Input: part model. Units: mm. Frame: model coordinates. Round coordinates to 2 decimals unless told otherwise and drop trailing zeros. Order: outer loops, then holes, each group sorted by start corner. A loop starts at its lowest first (then second) coordinate and runs counter-clockwise, first axis right, second up. Notation, with made-up numbers: M 27,84 L 58,84 A31 cw 58,118 Z; hole C -25.75,-29.75 d8. An arc over 180 degrees is marked long. One line per question, with ' | ' between items.
Autodesk Inventor part; units mm, degrees
ref_plane "YZ Plane" through (0, 0, 0) normal (1, 0, 0) x (0, 1, 0)
ref_plane "XZ Plane" through (0, 0, 0) normal (0, 1, 0) x (-1, 0, 0)
ref_plane "XY Plane" through (0, 0, 0) normal (0, 0, 1) x (1, 0, 0)
sketch "Esquisse1" plane through (0, 0, 0) normal (0, 0, 1) x (1, 0, 0)
  line L0 (22.3904, 80.6375) -> (22.3904, -39.3625)
  line L1 (-37.6096, 80.6375) -> (-37.6096, -39.3625)
  line L2 (-37.6096, -39.3625) -> (22.3904, -39.3625)
  line L3 (-37.6096, 80.6375) -> (22.3904, 80.6375)
  point P0 (0, 0)
  dimension "d0" = 120
  dimension "d1" = 60
extrude "Extrusion1" add sketch "Esquisse1" along normal mid plane 10
sketch "Esquisse2" plane through (22.3904, -39.3625, 5) normal (1, 0, 0) x (0, 0, -1)
  circle A0 centre (5, 100) radius 1.5
  line L0 (10, 0) -> (0, 0)
  point P0 (5, 39.3625)
  point P1 (5, 0)
  dimension "d10" = 100
  dimension "d11" = 3
sketch "Esquisse3" plane through (22.3904, -39.3625, 5) normal (1, 0, 0) x (0, 0, -1)
  circle A0 centre (5, 20) radius 1.5
  line L0 (10, 0) -> (0, 0)
  circle A1 centre (5, 100) radius 1.5
  point P0 (5, 39.3625)
  point P1 (5, 0)
  dimension "d4" = 20
  dimension "d5" = 3
  dimension "d6" = 100
  dimension "d7" = 3
extrude "Extrusion2" cut sketch "Esquisse3" against normal through all contours A0
extrude "Extrusion3" cut sketch "Esquisse2" against normal blind 60
properties part number "plaque de separation"
Item 1: Mould query, pull axis Z, two halves, no side actions, for faces 1 (the cylindrical face through (-7.19, 62.125, 0.195)), 2 (the flat face through (-8, 21, 5)), 3 (the flat face through (-8, 80.638, 0)), 4 (the flat face through (-8, 21, -5)). Classes: +Z half, -Z half, draft (parallel to the pull), parting line (faces both ways), or undercut.
Report:
face 1: undercut | face 2: +Z half | face 3: draft | face 4: -Z half
Item 2: Line query: line 1 along Y through (x, z) = (-13, 0). Output: solid intervals per line, ascending. Write a range as from..to.
Report:
line 1: -39.36..-20.86, -17.86..59.14, 62.14..80.64
Item 3: Section query A-A, the plane z = 0. Return loops of the section in (x, y), plus the area to 3 significant figures.
Report:
outline: M -37.61,-39.36 L 22.39,-39.36 L 22.39,-20.86 L -37.61,-20.86 Z; M -37.61,-17.86 L 22.39,-17.86 L 22.39,59.14 L -37.61,59.14 Z; M -37.61,62.14 L 22.39,62.14 L 22.39,80.64 L -37.61,80.64 Z | area: 6,840 mm²
